Could you check a few things on this model? Use its own coordinates, in mm. Give positions to 0.01 mm unless a question says otherwise; leave off trailing zeros. Write each loop counter-clockwise with the first axis right and the second up, starting at its lowest first coordinate (ties: lowest second). Pieces come first, ordered by that corner, then holes. Notation, with made-up numbers: (17, 83.25) - (31, 83.25) arc R20 ccw to (31, 117.25) - close; hole circle Ø1 at (-22.75, 72). An arc over 180 degrees is marked (long way). Answer as CSV lines item,"result". Start each with the question number.
Q1. Will this pin go through, and if not, where does the flat tip stop? pin 1 Ø2.5 at (x, z) = (-11.1, -92) entering from +Y.
Q2. Imagine slicing it at A-A on y = 0.4. List the corners of the cut face in (x, z) for me.
Q3. Imagine slicing it at B-B on z = -57. List the corners of the cut face in (x, y) for me.
Q4. If I drill on line 1 along Z through (x, y) = (-42.5, 0.6); line 2 along X through (y, z) = (0.4, -92); line 3 along X through (y, z) = (0.15, -45.5), over which ranges is the centre line in solid material (lowest first)?
Q5. Imagine slicing it at C-C on x = -11.1. List the corners of the cut face in (y, z) for me.
Q6. We'd pull the mould along Z, two halves only. Please class faces 1 (the face through (-11.1, 0.5, -90.3)), 2 (the face through (-23, 0, -46)): pulls with the +Z half, pulls with the -Z half, needs draft (parallel to the pull), parting line crosses it, or undercut.
Autodesk Inventor part; units mm, degrees
ref_plane "YZ Plane" through (0, 0, 0) normal (1, 0, 0) x (0, 1, 0)
ref_plane "XZ Plane" through (0, 0, 0) normal (0, 1, 0) x (-1, 0, 0)
ref_plane "XY Plane" through (0, 0, 0) normal (0, 0, 1) x (1, 0, 0)
sketch "Szkic1" plane through (0, 0, 0) normal (0, 1, 0) x (-1, 0, 0)
  line L0 (0, 0) -> (39, 0)
  line L1 (39, 0) -> (39, -92.5)
  line L2 (39, -92.5) -> (0, -92.5)
  line L3 (0, -92.5) -> (0, 0)
  line L4 (39, 0) -> (47.6, 0)
  line L5 (47.6, 0) -> (47.6, -29)
  line L6 (47.6, -29) -> (39, -29)
  line L7 (39, -29) -> (39, 0)
  line L8 (0, -46.25) -> (39, -46.25) construction
  line L9 (0, 0) -> (7.8, 0) construction
  line L10 (7.8, 0) -> (7.8, -5) construction
  line L11 (7.8, -5) -> (0, -5) construction
  line L12 (0, -5) -> (0, 0) construction
  line L13 (0, -92.5) -> (7.8, -92.5) construction
  line L14 (7.8, -92.5) -> (7.8, -87.5) construction
  line L15 (7.8, -87.5) -> (0, -87.5) construction
  line L16 (0, -87.5) -> (0, -92.5) construction
  line L17 (39, -92.5) -> (47.6, -92.5)
  line L18 (47.6, -92.5) -> (47.6, -78.25)
  line L19 (47.6, -78.25) -> (39, -78.25)
  line L20 (39, -78.25) -> (39, -92.5)
  line L21 (39, -92.5) -> (18, -92.5) construction
  line L22 (18, -92.5) -> (18, -29.5) construction
  line L23 (18, -29.5) -> (39, -29.5) construction
  line L24 (39, -29.5) -> (39, -92.5) construction
  circle A0 centre (47.7, -0.5) radius 1.7
  circle A1 centre (11.1, -0.5) radius 1.7
  circle A2 centre (47.7, -92) radius 1.7
  circle A3 centre (11.1, -92) radius 1.7
  point P0 (13.8, -33.8)
  point P1 (13.8, -58.7)
  dimension "d0" = 39
  dimension "d1" = 92.5
  dimension "d2" = 8.6
  dimension "d3" = 29
  dimension "d4" = 33.8
  dimension "d5" = 33.8
  dimension "d6" = 5
  dimension "d7" = 7.8
  dimension "d9" = 14.25
  dimension "d10" = 63
  dimension "d11" = 21
  dimension "d12" = 0.1
  dimension "d13" = 3.4
  dimension "d14" = 0.5
  dimension "d15" = 36.6
extrude "Plytka" add sketch "Szkic1" along normal blind 1 contours L0 A1 L1 L2 A3 L3 | L0 A1 | A3 L2 | L4 A0 L5 L6 L1 | L4 L5 A0 | L1 L19 L18 A2 L17 | A2 L18 L17 picked at (10.5661, -0.3857) picked at (10.6392, -91.3315) picked at (47.4739, -1.4428) picked at (47.4739, -91.0572)
extrude "Otwory" cut sketch "Szkic1" along normal up to surface (1 mm away) contours A1 L0 | L0 A1 | A3 L2 | L2 A3 | A0 L5 L4 | L4 L5 A0 | A2 L18 L17 | L17 L18 A2
sketch "Marginesy(Nie dotycza spodu plytki w strefie czujnika lini)" plane through (0, 1, 0) normal (0, 1, 0) x (1, 0, 0)
  line L0 (-47.6, 0) -> (-39, 0)
  line L1 (-39, 0) -> (-39, 2.4)
  line L2 (-39, 2.4) -> (-47.6, 2.4)
  line L3 (-47.6, 2.4) -> (-47.6, 0)
  line L4 (-46.0752, 0) -> (-12.7248, 0)
  line L5 (-47.6, 29) -> (-47.6, 2.1971)
  line L6 (-39, 78.25) -> (-39, 29)
  line L7 (-39, 0) -> (-16.9, 0)
  line L8 (-16.9, 0) -> (-16.9, 0.4)
  line L9 (-16.9, 0.4) -> (-39, 0.4)
  line L10 (-39, 0.4) -> (-39, 0)
  line L11 (0, 0) -> (0, 92.5)
  line L12 (-16.9, 0) -> (0, 0)
  line L13 (0, 0) -> (0, 2.4)
  line L14 (0, 2.4) -> (-16.9, 2.4)
  line L15 (-16.9, 2.4) -> (-16.9, 0)
  line L16 (0, 46.25) -> (-39, 46.25) construction
  line L17 (-47.6, 92.5) -> (-39, 92.5)
  line L18 (-39, 92.5) -> (-39, 90.1)
  line L19 (-39, 90.1) -> (-47.6, 90.1)
  line L20 (-47.6, 90.1) -> (-47.6, 92.5)
  line L21 (-46.0752, 92.5) -> (-12.7248, 92.5)
  line L22 (-39, 92.5) -> (-16.9, 92.5)
  line L23 (-16.9, 92.5) -> (-16.9, 92.1)
  line L24 (-16.9, 92.1) -> (-39, 92.1)
  line L25 (-39, 92.1) -> (-39, 92.5)
  line L26 (-16.9, 92.5) -> (0, 92.5)
  line L27 (0, 92.5) -> (0, 90.1)
  line L28 (0, 90.1) -> (-16.9, 90.1)
  line L29 (-16.9, 90.1) -> (-16.9, 92.5)
  arc A0 (-47.6, 90.3029) -> (-46.0752, 92.5) centre (-47.7, 92) ccw construction
  circle A1 centre (-47.7, 92) radius 2.85 construction
  arc A2 (-12.7248, 92.5) -> (-9.4752, 92.5) centre (-11.1, 92) ccw construction
  circle A3 centre (-11.1, 92) radius 2.85 construction
  arc A4 (-46.0752, 0) -> (-47.6, 2.1971) centre (-47.7, 0.5) ccw construction
  arc A5 (-9.4752, 0) -> (-12.7248, 0) centre (-11.1, 0.5) ccw construction
  circle A6 centre (-47.7, 0.5) radius 2.85 construction
  circle A7 centre (-11.1, 0.5) radius 2.85 construction
  point P0 (0, 92.5)
  dimension "d20" = 2.4
  dimension "d21" = 0.4
  dimension "d22" = 22.1
  dimension "d24" = 5.7
properties part number "PlytkaWymiary"
Conclusion:
1,pin 1,"through"
2,outline,"(-47.6, -90.3) arc R1.7 cw to (-46.08, -92.5) - (-12.72, -92.5) arc R1.7 cw (long way) to (-9.48, -92.5) - (0, -92.5) - (0, 0) - (-9.48, 0) arc R1.7 cw (long way) to (-12.72, 0) - (-46.08, 0) arc R1.7 cw to (-47.6, -2.2) - (-47.6, -29) - (-39, -29) - (-39, -78.25) - (-47.6, -78.25) - close"
3,outline,"(-39, 0) - (0, 0) - (0, 1) - (-39, 1) - close"
4,line 1,"-92.5 to -78.25, -29 to 0"
4,line 2,"-46 to -12.8, -9.4 to 0"
4,line 3,"-39 to 0"
5,outline,"(0, -90.3) - (1, -90.3) - (1, -2.2) - (0, -2.2) - close"
6,face 1,"undercut"
6,face 2,"needs draft"
